Read the model definition and answer for the solid it produces. Units are mm, in the model's axes. A direction names the side the tool comes from. Coordinates: 2 decimals unless noted, no trailing zeros. Write each loop counter-clockwise with the first axis right and the second up, starting at its lowest first coordinate (ties: lowest second). Pieces come first, ordered by that corner, then holes.
from build123d import *

# Parameters (mm, degrees)
SKIZZE1_W                       = 34.00858099
SKIZZE1_H                       = 51.467136578
AUFSATZ_LINEAR_AUSTRAGEN1_DEPTH = 2
SKIZZE6_W                       = 10
SKIZZE6_H                       = 2
AUFSATZ_LINEAR_AUSTRAGEN2_DEPTH = 2
SKIZZE7_W                       = 2
SKIZZE7_H                       = 10
SCHNITT_LINEAR_AUSTRAGEN1_DEPTH = 2
SKIZZE8_W                       = 2
SKIZZE8_H                       = 10
SCHNITT_LINEAR_AUSTRAGEN2_DEPTH = 2


with BuildPart() as part:
    # Skizze1 → Aufsatz-Linear austragen1 (new body)
    with BuildSketch(Plane.XY):
        Rectangle(SKIZZE1_W, SKIZZE1_H)
    extrude(amount=AUFSATZ_LINEAR_AUSTRAGEN1_DEPTH)

    # Skizze6 → Aufsatz-Linear austragen2 (add)
    with BuildSketch(Plane.XZ.offset(25.733568289)):
        with Locations((0.286784859, 1)):
            Rectangle(SKIZZE6_W, SKIZZE6_H)
    extrude(amount=AUFSATZ_LINEAR_AUSTRAGEN2_DEPTH)

    # Skizze7 → Schnitt-Linear austragen1 (cut)
    with BuildSketch(Plane.ZY.offset(17.004290495)):
        with Locations((1, 10.733568289)):
            Rectangle(SKIZZE7_W, SKIZZE7_H)
    extrude(amount=-SCHNITT_LINEAR_AUSTRAGEN1_DEPTH, mode=Mode.SUBTRACT)

    # Skizze8 → Schnitt-Linear austragen2 (cut)
    with BuildSketch(Plane.ZY.offset(17.004290495)):
        with Locations((1, -9.266431711)):
            Rectangle(SKIZZE8_W, SKIZZE8_H)
    extrude(amount=-SCHNITT_LINEAR_AUSTRAGEN2_DEPTH, mode=Mode.SUBTRACT)


solid = part.part
Item 1: Determine the mould class of faces 1 (the flat face through (-15.004, -9, 1)), 2 (the flat face through (-17.004, -20, 1)), 3 (the flat face through (0, 25.734, 1)) for opening direction Y: +Y half, -Y half, draft (parallel to the pull), parting line (faces both ways), or undercut.
Item 2: The part is cut by section B-B (x = 10). Give the vertices of the cut face in (y, z), and give its area (3 significant figures).
Item 3: For faces 4 (the flat face through (-11, -25.734, 1)), 5 (the flat face through (5.287, -27, 1)), 6 (the flat face through (-16, -14.266, 1)), determine the directions among +Z, -Z, +X, -X, +Y, -Y from which every point of the face is accessible in a straight line to the end or side of a thin tool.
Item 4: Given pin 1 (0.6 mm diameter, centred on x = -14, z = 0.5, fed in from -Y); pin 2 (0.6 mm diameter, centred on y = 8.5, z = 1.5, fed in from -X); pin 3 (0.6 mm diameter, centred on y = -27, z = 1, fed in from +X), each flat-ended and moving along its own axis, determine where each tip first touches the part or whether it passes through.
Item 5: Find the intervals of material crossed by probe 1 along X at (y, z) = (-12.5, 0.1); probe 2 along Y at (x, z) = (-7, 0.35), in increasing order.
Item 6: The part is cut by section A-A (z = 1.6). Give the vertices of the cut face in (x, y), and give its area (3 significant figures).
Answer:
1. face 1: undercut
1. face 2: draft
1. face 3: +Y half
2. outline: (-25.73, 0) - (25.73, 0) - (25.73, 2) - (-25.73, 2) - close
2. area: 103 mm2
3. face 4: +Z, -Z, -X, -Y
3. face 5: +Z, -Z, +X, -Y
3. face 6: +Z, -Z, -X
4. pin 1: stops at y = -25.73
4. pin 2: stops at x = -15
4. pin 3: stops at x = 5.29
5. probe 1: x = -15 to 17
5. probe 2: y = -25.73 to 25.73
6. outline: (-17, -25.73) - (-4.71, -25.73) - (-4.71, -27.73) - (5.29, -27.73) - (5.29, -25.73) - (17, -25.73) - (17, 25.73) - (-17, 25.73) - (-17, 15.73) - (-15, 15.73) - (-15, 5.73) - (-17, 5.73) - (-17, -4.27) - (-15, -4.27) - (-15, -14.27) - (-17, -14.27) - close
6. area: 1,730 mm2
